```python
from build123d import *

# Parameters (mm, degrees)
SKETCH1_R           = 20
SKETCH1_R_2         = 1.5
BOSS_EXTRUDE1_DEPTH = 7


with BuildPart() as part:
    # Sketch1 → Boss-Extrude1 (new body)
    with BuildSketch(Plane.XY):
        with BuildLine():
            Line((77.735606869, -1.559100202), (77.735606869, 1.559100202))
            ThreePointArc((77.735606869, 1.559100202), (77.170867479, 2.951948716), (75.795579887, 3.558200809))
            Line((75.795579887, 3.558200809), (27.735606869, 5))
            ThreePointArc((27.735606869, 5), (25.240316673, 5.865195462), (23.685438565, 8))
            ThreePointArc((23.685438565, 8), (-25, 0), (23.685438565, -8))
            ThreePointArc((23.685438565, -8), (25.240316673, -5.865195462), (27.735606869, -5))
            Line((27.735606869, -5), (75.795579887, -3.558200809))
            ThreePointArc((75.795579887, -3.558200809), (77.170867479, -2.951948716), (77.735606869, -1.559100202))
        make_face()
        Circle(SKETCH1_R, mode=Mode.SUBTRACT)
        with Locations((74.127359446, 0)):
            Circle(SKETCH1_R_2, mode=Mode.SUBTRACT)
    extrude(amount=BOSS_EXTRUDE1_DEPTH)


solid = part.part
```
CAD build for the part. Positions are in the model's coordinates, mm. Round coordinates to 2 decimals unless told otherwise and drop trailing zeros. Write each loop counter-clockwise with the first axis right and the second up, starting at its lowest first coordinate (ties: lowest second). Pieces come first, ordered by that corner, then holes. Notation, with made-up numbers: (-26, 71.5) - (-13, 71.5) arc R25 cw to (-13, 91.5) - close; hole circle Ø7 at (30.5, -32). An arc over 180 degrees is marked (long way). Return JSON: item names as keys, results as strings. Group by question number.
Item 1: Mould opens along X. For faces 1 (the face through (-24.98, 0.99, 3.45)), 2 (the face through (25.271, 5.843, 3.451)), 3 (the face through (-4.336, -19.524, 3.451)) say: +X half, -X half, draft (parallel to the pull), parting line (faces both ways), or undercut.
Item 2: Band-saw the part on C-C on y = 0. List the corners of the cut face in (x, z).
Item 3: Band-saw the part on B-B on z = 4.75. List the corners of the cut face in (x, y).
Item 4: Probe probe 1 along Y at (x, z) = (0, 3.25); probe 2 along Y at (x, z) = (-18, 6); probe 3 along X at (y, z) = (2, 3.25). List the from-to ranges inside material, lowest first.
Item 5: Flat gauge pins, fed straight in: pin 1 Ø3 at (y, z) = (-16, 6) entering from -X; pin 2 Ø2 at (y, z) = (10, 4) entering from +X; pin 3 Ø3 at (x, z) = (59.5, 2) entering from +Y; pin 4 Ø3.5 at (x, y) = (74.13, 0) entering from -Z. Where does each tip first touch, or does it go through?
Item 6: Band-saw the part on A-A on x = 0. List the corners of the cut face in (y, z), plus the area to 3 significant figures.
Item 7: Band-saw the part on D-D on y = -17. List the corners of the cut face in (x, z), plus the area to 3 significant figures.
Resolved:
{
 "1": {"face 1": "parting line", "face 2": "+X half", "face 3": "undercut"},
 "2": {"outline": "(-25, 0) - (-20, 0) - (-20, 7) - (-25, 7) - close; (20, 0) - (72.63, 0) - (72.63, 7) - (20, 7) - close; (75.63, 0) - (77.74, 0) - (77.74, 7) - (75.63, 7) - close"},
 "3": {"outline": "(23.69, -8) arc R4.41 cw to (27.74, -5) - (75.8, -3.56) arc R2 ccw to (77.74, -1.56) - (77.74, 1.56) arc R2 ccw to (75.8, 3.56) - (27.74, 5) arc R4.41 cw to (23.69, 8) arc R25 ccw (long way) to start; hole circle Ø40 at (0, 0); hole circle Ø3 at (74.13, 0)"},
 "4": {"probe 1": "y = -25 to -20, 20 to 25", "probe 2": "y = -17.35 to -8.72, 8.72 to 17.35", "probe 3": "x = -24.92 to -19.9, 19.9 to 77.69"},
 "5": {"pin 1": "stops at x = -20.37", "pin 2": "stops at x = 23.32", "pin 3": "stops at y = 4.09", "pin 4": "stops at z = 0"},
 "6": {"outline": "(-25, 0) - (-20, 0) - (-20, 7) - (-25, 7) - close; (20, 0) - (25, 0) - (25, 7) - (20, 7) - close", "area": "70.0 mm²"},
 "7": {"outline": "(-18.33, 0) - (-10.54, 0) - (-10.54, 7) - (-18.33, 7) - close; (10.54, 0) - (18.33, 0) - (18.33, 7) - (10.54, 7) - close", "area": "109 mm²"}
}
